from build123d import *

# Parameters (mm, degrees)
F0_W      = 34.420416
F0_H      = 28.010136
F1_DEPTH  = 25.4
F2_W      = 21.713977
F2_H      = 10.812225
F3_DEPTH  = 5.08
F4_W      = 32.364089
F4_H      = 25.274814
F5_DEPTH  = 3.81
F6_W      = 11.602566
F6_H      = 21.341514
F7_DEPTH  = 15.24
F8_W      = 10.458534
F8_H      = 6.296051
F9_DEPTH  = 5.08
F10_W     = 5.08
F10_H     = 6.296051
F11_DEPTH = 25.4


with BuildPart() as f1:
    # F0 (on Front) → F1 (new body)
    with BuildSketch(Plane.XZ):
        Polygon((45.290023, 17.697947), (-39.297804, 17.697947), (-39.297804, -23.968874), (45.290023, -23.968874), (45.290023, -10.312189), align=None)
        with Locations((62.500231, 3.692879)):
            Rectangle(F0_W, F0_H)
    extrude(amount=F1_DEPTH)

    # F2 (on face) → F3 (join)
    with BuildSketch(Plane.XZ.offset(25.4)):
        with Locations((-13.639831, 7.048171)):
            Rectangle(F2_W, F2_H)
    extrude(amount=F3_DEPTH)

    # F4 (on face) → F5 (cut)
    with BuildSketch(Plane.XZ.offset(25.4)):
        with Locations((62.433859, 3.767056)):
            Rectangle(F4_W, F4_H)
    extrude(amount=-F5_DEPTH, mode=Mode.SUBTRACT)

    # F6 (on face) → F7 (join)
    with BuildSketch(Plane.XZ.offset(25.4)):
        with Locations((33.965688, 3.841953)):
            Rectangle(F6_W, F6_H)
    extrude(amount=F7_DEPTH)

    # F8 (on face) → F9 (cut)
    with BuildSketch(Plane.YZ.offset(39.766971)):
        with Locations((-30.629267, 4.275792)):
            Rectangle(F8_W, F8_H)
    extrude(amount=-F9_DEPTH, mode=Mode.SUBTRACT)

    # F10 (on face) → F11 (cut)
    with BuildSketch(Plane.XZ.offset(25.4)):
        with Locations((37.226971, 4.275792)):
            Rectangle(F10_W, F10_H)
    extrude(amount=-F11_DEPTH, mode=Mode.SUBTRACT)


solid = f1.part
Input: part model. Units: mm. Frame: model coordinates. A direction names the side the tool comes from. Coordinates: 2 decimals unless noted, no trailing zeros. Write each loop counter-clockwise with the first axis right and the second up, starting at its lowest first coordinate (ties: lowest second). Pieces come first, ordered by that corner, then holes. Notation, with made-up numbers: M 78.25,21.25 L 113.25,21.25 A16 ccw 113.25,30.25 Z; hole C 3,-32 d8. An arc over 180 degrees is marked long. Answer as a JSON object with one key per item and string values. Group by question number.
(1) Section D-D on y = -10. Output: boundary loops of the cut face in (x, z).
(2) Section C-C on z = 11. Output: boundary loops of the cut face in (x, y), plus the area to 3 significant figures.
(3) Ray query, line 1 along X through (y, z) = (-24, -1); line 2 along Z through (x, y) = (39, -15.5); line 3 along X through (y, z) = (-38, -3). Return the intervals inside material, ascending. Write a range as [from, to].
(4) Mould query, pull axis Z, two halves, no side actions, for faces 4 (the face through (-39.298, -13, -3)), 5 (the face through (62, -21.59, 4)), 6 (the face through (34, -33, 14.513)). Classes: pulls with the +Z half, pulls with the -Z half, needs draft (parallel to the pull), parting line crosses it, or undercut.
(5) Section A-A on y = -28. Output: boundary loops of the cut face in (x, z), plus the area to 3 significant figures.
(6) Set-up query: faces 1 (the face through (-2.783, -28, 7)), 2 (the face through (-14, -28, 1.642)), 3 (the face through (62, -13, -10.312)). Return all of +Z, -Z, +X, -X, +Y, -Y with unobstructed straight access to the full face (end or side cutting, diameter ignored); none if empty.
(7) Contact query for flat-ended pins moving along their axis: P1, Ø1.9, axis at y = -27, z = 3, coming from the +X side; P2, Ø4, axis at x = 62, y = -23, coming from the -Z side; P3, Ø3.5, axis at x = 32.5, y = -31.5, coming from the -Z side. Output: stop coordinate, or through.
(8) Section B-B on x = -9. Output: boundary loops of the cut face in (y, z), plus the area to 3 significant figures.
Result set:
{
 "1": {"outline": "M -39.3,-23.97 L 45.29,-23.97 L 45.29,-10.31 L 79.71,-10.31 L 79.71,17.7 L -39.3,17.7 Z; hole M 34.69,1.13 L 39.77,1.13 L 39.77,7.42 L 34.69,7.42 Z"},
 "2": {"outline": "M -39.3,-25.4 L -24.5,-25.4 L -24.5,-30.48 L -2.78,-30.48 L -2.78,-25.4 L 28.16,-25.4 L 28.16,-40.64 L 39.77,-40.64 L 39.77,-25.4 L 46.25,-25.4 L 46.25,-21.59 L 78.62,-21.59 L 78.62,-25.4 L 79.71,-25.4 L 79.71,0 L -39.3,0 Z", "area": "3,190 mm2"},
 "3": {"line 1": "x = [-39.3, 46.25], [78.62, 79.71]", "line 2": "z = [-23.97, 1.13], [7.42, 17.7]", "line 3": "x = [28.16, 39.77]"},
 "4": {"face 4": "needs draft", "face 5": "undercut", "face 6": "pulls with the +Z half"},
 "5": {"outline": "M -24.5,1.64 L -2.78,1.64 L -2.78,12.45 L -24.5,12.45 Z; M 28.16,-6.83 L 39.77,-6.83 L 39.77,1.13 L 34.69,1.13 L 34.69,7.42 L 39.77,7.42 L 39.77,14.51 L 28.16,14.51 Z", "area": "450 mm2"},
 "6": {"face 1": "+Z, -Z, -Y", "face 2": "-Z, -X, -Y", "face 3": "-Z, +X, +Y, -Y"},
 "7": {"P1": "stops at x = 34.69", "P2": "stops at z = -10.31", "P3": "stops at z = -6.83"},
 "8": {"outline": "M -30.48,1.64 L -25.4,1.64 L -25.4,-23.97 L 0,-23.97 L 0,17.7 L -25.4,17.7 L -25.4,12.45 L -30.48,12.45 Z", "area": "1,110 mm2"}
}
